from build123d import *

# Parameters (mm, degrees)
SKETCH_W        = 31.75
SKETCH_H        = 31.75
SKETCH_W_2      = 26.2128
SKETCH_H_2      = 26.2128
PAD_DEPTH       = 777.09014
POCKET_DEPTH    = 31.75
POCKET001_DEPTH = 31.75


with BuildPart() as part:
    # Sketch → Pad (new body)
    with BuildSketch(Plane.XY):
        Rectangle(SKETCH_W, SKETCH_H)
        Rectangle(SKETCH_W_2, SKETCH_H_2, mode=Mode.SUBTRACT)
    extrude(amount=PAD_DEPTH)

    # Sketch001 → Pocket (cut)
    with BuildSketch(Plane.XZ.offset(15.875)):
        Polygon((15.875, 0), (-15.875, 0), (-15.875, 6.349981), align=None)
    extrude(amount=-POCKET_DEPTH, mode=Mode.SUBTRACT)

    # Sketch002 → Pocket001 (cut)
    with BuildSketch(Plane.XZ.offset(15.875)):
        Polygon((15.875, 777.09014), (-15.875, 777.09014), (-15.875, 751.061397), align=None)
    extrude(amount=-POCKET001_DEPTH, mode=Mode.SUBTRACT)


solid = part.part
Source: CAD feature listing. Evaluate the final solid. Frame: model axes, mm. A direction names the side the tool comes from. Round coordinates to 2 decimals unless told otherwise and drop trailing zeros. Order: outer loops, then holes, each group sorted by start corner. A loop starts at its lowest first (then second) coordinate and runs counter-clockwise, first axis right, second up. Notation, with made-up numbers: (46.25, -15.5) -> (104.25, -15.5) arc R27 cw to (104.25, 20.5) -> close; hole circle Ø7 at (3, -21.5). An arc over 180 degrees is marked (long way). Answer as CSV lines item,"result".
Item 1: Section B-B, the plane z = 516. Return loops of the section in (x, y) (3 decimals), plus the area to 3 significant figures.
A:
outline,"(-15.875, -15.875) -> (15.875, -15.875) -> (15.875, 15.875) -> (-15.875, 15.875) -> close; hole (-13.106, -13.106) -> (13.106, -13.106) -> (13.106, 13.106) -> (-13.106, 13.106) -> close"
area,"321 mm²"
Item 2: Line query: L1, parallel to X at y = 7.5, z = 436 (3 decimals); L2, parallel to Z at x = -13.5, y = 5. Output: solid intervals per line, ascending.
A:
L1,"-15.875 to -13.106, 13.106 to 15.875"
L2,"5.87 to 753.01"
Item 3: Pin query (flat end, axial travel): pin 1 Ø12 at (x, y) = (7.5, 10) entering from +Z; pin 2 Ø4 at (x, y) = (9.5, 10) entering from -Z (1 decimal); pin 3 Ø10 at (x, y) = (-2, -11.5) entering from -Z. Return the tip coordinate at first contact, or that it passes through.
A:
pin 1,"z = 775.14"
pin 2,"through"
pin 3,"z = 2.63"
Item 4: Section A-A, the plane y = 7. Return loops of the section in (x, z) (3 decimals), plus the area to 3 significant figures.
A:
outline,"(-15.875, 6.35) -> (-13.106, 5.796) -> (-13.106, 753.331) -> (-15.875, 751.061) -> close; (13.106, 0.554) -> (15.875, 0) -> (15.875, 777.09) -> (13.106, 774.82) -> close"
area,"4,210 mm²"
Item 5: Reachability of faces 5 (the face through (0, -13.106, 382)), 6 (the face through (-0.222, 13.889, 763.894)) from +Z, -Z, +X, -X, +Y, -Y: full face, straight path, thin tool, end or side. Return the list, or none.
A:
face 5,"+Z, -Z"
face 6,"+Z, -X, +Y, -Y"
Item 6: Pull-direction query (Y, two-part tool) for faces 1 (the face through (0, 13.106, 382)), 2 (the face through (0, -15.875, 383)), 3 (the face through (-0.22, 13.89, 3.22)), 4 (the face through (0, 15.875, 383)); classes: pulls with the +Y half, pulls with the -Y half, needs draft (parallel to the pull), parting line crosses it, or undercut.
A:
face 1,"undercut"
face 2,"pulls with the -Y half"
face 3,"needs draft"
face 4,"pulls with the +Y half"
Item 7: Section C-C, the plane x = -8. Return loops of the section in (y, z) (3 decimals).
A:
outline,"(-15.875, 4.775) -> (-13.106, 4.775) -> (-13.106, 757.517) -> (-15.875, 757.517) -> close; (13.106, 4.775) -> (15.875, 4.775) -> (15.875, 757.517) -> (13.106, 757.517) -> close"
